Can you work these out from the model? Positions are in its coordinate system, mm. Face numbers are marked on the shaded views. Round coordinates to 2 decimals unless told otherwise and drop trailing zeros. Write each loop counter-clockwise with the first axis right and the second up, starting at its lowest first coordinate (ties: lowest second). Pieces come first, ordered by that corner, then holes. Notation, with made-up numbers: M 25.25,34.25 L 61.25,34.25 A24 cw 61.25,66.25 Z; hole C 11,81 d11. An arc over 180 degrees is marked long. Answer in a Markdown table with one row per item. Add a question column.
(1) Suppose I cut it at B-B, the plane y = 6. Write out the boundary of the cut face in (x, z).
(2) I'm going to push flat-ended pins straight in: pin 1 (4 mm diameter, centred on x = 25, y = -18.5, fed in from -Z); pin 2 (25 mm diameter, centred on x = 0, y = 0, fed in from +Z); pin 3 (3 mm diameter, centred on y = 10, z = 2.5, fed in from -X). Where does each tip first touch, or does it pass through?
(3) If I drill on probe 1 along Y at (x, z) = (0, 5.4); probe 2 along X at (y, z) = (-5.5, 2.25); probe 3 along X at (y, z) = (11, 5.75), over which ranges is the centre line in solid material (lowest first)?
(4) Suppose I cut it at D-D, the plane x = -14.5. Write out the boundary of the cut face in (y, z).
(5) If we mould it in two halves opening along X, with no side actions, what happens to the marked faces 1, 2 and 3? For each: released by +X, released by -X, zero draft, split by the parting line, or undercut.
(6) Suppose I cut it at C-C, the plane z = 1.75. Count the separate pieces of the cut face and the enclosed holes in it, then the cut area to 3 significant figures.
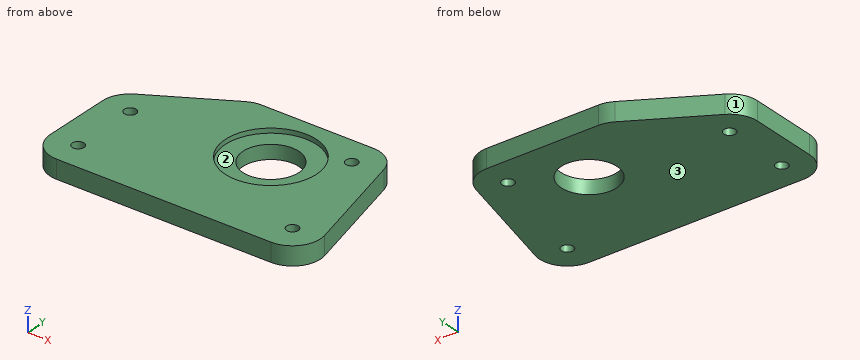
from build123d import *

# Parameters (mm, degrees)
SKETCH1_R                  = 9.525
BOSS_EXTRUDE1_DEPTH        = 6.35
SKETCH6_R                  = 15.5702
CUT_EXTRUDE2_DEPTH         = 1.5875
TAP_DRILL_FOR_10_32_TAP1_D = 4.0386


with BuildPart() as part:
    # Sketch1 → Boss-Extrude1 (new body)
    with BuildSketch(Plane.XY):
        with BuildLine():
            Line((-45.162617117, -36.5125), (28.303378868, -36.5125))
            ThreePointArc((28.303378868, -36.5125), (35.784732944, -32.882834273), (37.564288704, -24.760130697))
            Line((37.564288704, -24.760130697), (28.400743011, 13.339869303))
            ThreePointArc((28.400743011, 13.339869303), (25.035167449, 18.593854076), (19.139833175, 20.6375))
            Line((19.139833175, 20.6375), (-19.139833175, 20.6375))
            ThreePointArc((-19.139833175, 20.6375), (-21.60508458, 20.312943495), (-23.902333175, 19.361391971))
            Line((-23.902333175, 19.361391971), (-49.925117117, 4.337130657))
            ThreePointArc((-49.925117117, 4.337130657), (-53.411509088, 0.850738686), (-54.687617117, -3.911761314))
            Line((-54.687617117, -3.911761314), (-54.687617117, -26.9875))
            ThreePointArc((-54.687617117, -26.9875), (-51.897809208, -33.722692091), (-45.162617117, -36.5125))
        make_face()
        Circle(SKETCH1_R, mode=Mode.SUBTRACT)
    extrude(amount=BOSS_EXTRUDE1_DEPTH)

    # Sketch6 → Cut-Extrude2 (cut)
    with BuildSketch(Plane.XY.offset(6.35)):
        Circle(SKETCH6_R)
    extrude(amount=-CUT_EXTRUDE2_DEPTH, mode=Mode.SUBTRACT)

    # Tap Drill for #10-32 Tap1 (through all)
    with Locations(Plane(origin=(0, 0, 0), x_dir=(-1, 0, 0), z_dir=(0, 0, -1))):
        with Locations((-28.303378868, -26.9875), (-19.139833175, 11.1125), (45.162617117, -3.911761314), (45.162617117, -26.9875)):
            Hole(TAP_DRILL_FOR_10_32_TAP1_D / 2)


solid = part.part
Calculated:
| question | item | result |
|---|---|---|
| 1 | outline | M -47.04,0 L -7.4,0 L -7.4,4.76 L -14.37,4.76 L -14.37,6.35 L -47.04,6.35 Z; M 7.4,0 L 30.17,0 L 30.17,6.35 L 14.37,6.35 L 14.37,4.76 L 7.4,4.76 Z |
| 2 | pin 1 | z = 0 |
| 2 | pin 2 | z = 4.76 |
| 2 | pin 3 | x = -42.71 |
| 3 | probe 1 | -36.51 to -15.57, 15.57 to 20.64 |
| 3 | probe 2 | -54.69 to -46.41, -43.92 to -7.78, 7.78 to 32.93 |
| 3 | probe 3 | -38.38 to -11.02, 11.02 to 17.12, 21.16 to 28.96 |
| 4 | outline | M -36.51,0 L 20.64,0 L 20.64,6.35 L 5.67,6.35 L 5.67,4.76 L -5.67,4.76 L -5.67,6.35 L -36.51,6.35 Z |
| 5 | face 1 | released by -X |
| 5 | face 2 | undercut |
| 5 | face 3 | zero draft |
| 6 | separate pieces | 1 |
| 6 | enclosed holes | 5 |
| 6 | area | 4,320 mm² |
